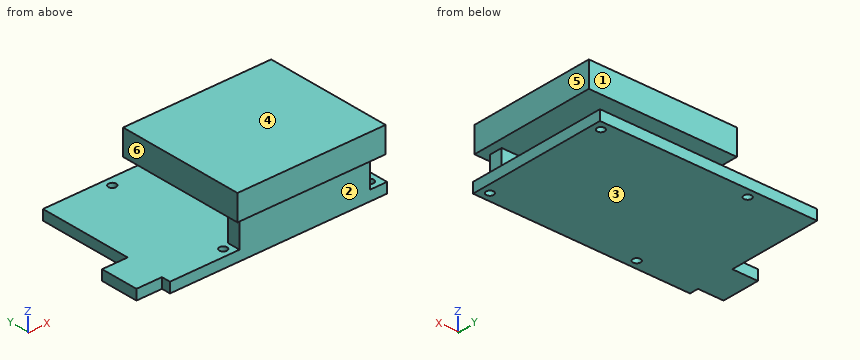
from build123d import *

# Parameters (mm, degrees)
F0_R     = 1.5
F0_W     = 10
F0_H     = 15
F1_DEPTH = 4
F2_W     = 51
F2_H     = 5
F3_DEPTH = 12
F4_W     = 58
F4_H     = 50
F5_DEPTH = 10


with BuildPart() as f1:
    # F0 (on Top) → F1 (new body)
    with BuildSketch(Plane.XY):
        Polygon((42.5, 27.75), (-42.5, 27.75), (-42.5, -9.25), (-42.5, -24.25), (-42.5, -27.75), (42.5, -27.75), align=None)
        with Locations((-18.5, -24.25)):
            Circle(F0_R, mode=Mode.SUBTRACT)
        with Locations((39, -24.25)):
            Circle(F0_R, mode=Mode.SUBTRACT)
        with Locations((-18.5, 24.25)):
            Circle(F0_R, mode=Mode.SUBTRACT)
        with Locations((39, 24.25)):
            Circle(F0_R, mode=Mode.SUBTRACT)
        with Locations((-47.5, -16.75)):
            Rectangle(F0_W, F0_H)
    extrude(amount=F1_DEPTH)

    # F2 (on face) → F3 (join)
    with BuildSketch(Plane.XY.offset(4)):
        with Locations((10.25, -25.25)):
            Rectangle(F2_W, F2_H)
    extrude(amount=F3_DEPTH)

    # F4 (on face) → F5 (join)
    with BuildSketch(Plane.XY.offset(16)):
        with Locations((10.25, -5.75)):
            Rectangle(F4_W, F4_H)
    extrude(amount=F5_DEPTH)


solid = f1.part
The listing builds one solid part. Answer for the finished solid, in the listing's coordinates (mm). Face numbers are marked on the shaded views. A direction names the side the tool comes from. Coordinates: 2 decimals unless noted, no trailing zeros. Write each loop counter-clockwise with the first axis right and the second up, starting at its lowest first coordinate (ties: lowest second). Pieces come first, ordered by that corner, then holes. Notation, with made-up numbers: (57, 55.5) - (89, 55.5) arc R10 cw to (89, 70.5) - close; hole circle Ø8 at (-7.5, 55). An arc over 180 degrees is marked (long way). Return JSON: item names as keys, results as strings.
1. For a pull along Y with two mould halves and no side action, classify the marked faces 1, 2 and 3 as +Y half, -Y half, draft (parallel to the pull), parting line (faces both ways), or undercut.
Final values:
{"face 1": "+Y half", "face 2": "-Y half", "face 3": "draft"}
2. The part is cut by section C-C on x = 29. Determine the outline of the cut face in (y, z), then the cut area to 3 significant figures.
Final values:
{"outline": "(-30.75, 16) - (-27.75, 16) - (-27.75, 0) - (27.75, 0) - (27.75, 4) - (-22.75, 4) - (-22.75, 16) - (19.25, 16) - (19.25, 26) - (-30.75, 26) - close", "area": "782 mm^2"}
3. Which of the six approach directions +Z, -Z, +X, -X, +Y, -Y give full straight-line access (tool end or side, diameter ignored) to the marked faces 4, 5 and 6?
Final values:
{"face 4": "+Z, +X, -X, +Y, -Y", "face 5": "+Z, +X, +Y, -Y", "face 6": "+Z, -X, +Y, -Y"}
4. The part is cut by section B-B on y = -19.5. Determine the outline of the cut face in (x, z), then the cut area to 3 significant figures.
Final values:
{"outline": "(-52.5, 0) - (42.5, 0) - (42.5, 4) - (-52.5, 4) - close; (-18.75, 16) - (39.25, 16) - (39.25, 26) - (-18.75, 26) - close", "area": "960 mm^2"}
5. The part is cut by section D-D on z = 19.25. Determine the outline of the cut face in (x, y).
Final values:
{"outline": "(-18.75, -30.75) - (39.25, -30.75) - (39.25, 19.25) - (-18.75, 19.25) - close"}
6. The part is cut by section A-A on y = 24.25. Determine the outline of the cut face in (x, z), then the cut area to 3 significant figures.
Final values:
{"outline": "(-42.5, 0) - (-20, 0) - (-20, 4) - (-42.5, 4) - close; (-17, 0) - (37.5, 0) - (37.5, 4) - (-17, 4) - close; (40.5, 0) - (42.5, 0) - (42.5, 4) - (40.5, 4) - close", "area": "316 mm^2"}
7. Consider line 1 along Y through (x, z) = (-18.5, 2.5); line 2 along Z through (x, y) = (-2, 16); line 3 along X through (y, z) = (-23, 1.5). Determine where each line is inside the solid, lowest interval first.
Final values:
{"line 1": "-27.75 to -25.75, -22.75 to 22.75, 25.75 to 27.75", "line 2": "0 to 4, 16 to 26", "line 3": "-52.5 to -19.33, -17.67 to 38.17, 39.83 to 42.5"}
8. Each of these flat-tipped pins is pushed along its axis until it touches: pin 1 Ø12 at (y, z) = (21.5, 6) entering from -X; pin 2 Ø5 at (y, z) = (-17.5, 21) entering from +X; pin 3 Ø1.5 at (y, z) = (-26, 10.5) entering from +X; pin 4 Ø4 at (x, y) = (26.5, -1) entering from -Z. Where does it stop, or does it pass through?
Final values:
{"pin 1": "x = -42.5", "pin 2": "x = 39.25", "pin 3": "x = 35.75", "pin 4": "z = 0"}
